```python
from build123d import *
from build123d.topology import SkipClean

# Parameters (mm, degrees)
SKETCH1_R            = 1.25
BRACKET_DEPTH        = 7.6
SKETCH2_R            = 1.5
ARM_DEPTH            = 1.6
SKETCH3_R            = 1.25
MOUNT_BLIND_DEPTH    = 1
EFFECTOR_START       = -5
SKETCH4_R            = 4
SKETCH4_R_2          = 1.5
EFFECTOR_MOUNT_DEPTH = 5
MOUNT_TRAP_DEPTH     = 2.4
SKETCH6_R            = 1.5
MOUNT_ADAPTOR_DEPTH  = 2.4
SKETCH7_W            = 12.99999996
SKETCH7_H            = 31.965
MIRROR_DELETE_DEPTH  = 37.150933583
ARM_SUPPORT_DEPTH    = 1.4
BODY_CHAMFER_SIZE    = 0.5
ARM_FILLET_R         = 0.5


with BuildPart() as part:
    # Sketch1 → Bracket (new body)
    with BuildSketch(Plane(origin=(0, 0, 0), x_dir=(1, 0, 0), z_dir=(0, 1, 0))):
        with BuildLine():
            Line((0, 7.765), (-9.4, 7.765))
            Line((-9.4, 7.765), (-12.531403257, 1.878614127))
            ThreePointArc((-12.531403257, 1.878614127), (-12.99999996, 0), (-12.531403257, -1.878614127))
            Line((-12.531403257, -1.878614127), (-9.4, -7.765))
            Line((-9.4, -7.765), (0, -7.765))
            Line((0, -7.765), (0, -5.765))
            ThreePointArc((0, -5.765), (-5.765, 0), (0, 5.765))
            Line((0, 5.765), (0, 7.765))
        make_face()
        with Locations(Location((-9, 0, 0), (0, 0, 90))):
            Circle(SKETCH1_R, mode=Mode.SUBTRACT)
    bracket = extrude(amount=BRACKET_DEPTH)

    # Sketch2 → Arm (add)
    with BuildSketch(Plane(origin=(-6.4, 0, 0), x_dir=(0, 0, -1), z_dir=(1, 0, 0))):
        with BuildLine():
            Line((-7.765, 0), (18.162978801, -15.342462002))
            ThreePointArc((18.162978801, -15.342462002), (24.160405232, -12.461418203), (19.2, -8.027016654))
            Line((19.2, -8.027016654), (7.765, 0))
            Line((7.765, 0), (-7.765, 0))
        make_face()
        with Locations((20.2, -11.9)):
            Circle(SKETCH2_R, mode=Mode.SUBTRACT)
    arm = extrude(amount=-ARM_DEPTH)

    # Sketch3 → Mount Blind (add)
    with BuildSketch(Plane.XZ):
        with Locations(Location((-9, 0, 0), (0, 0, 270))):
            Circle(SKETCH3_R)
    mount_blind = extrude(amount=-MOUNT_BLIND_DEPTH)

    # Sketch4 → Effector Mount (add)
    with SkipClean():  # the faces are left unmerged after this step: merging them gives an invalid solid
        with BuildSketch(Plane.ZY.offset(8).offset(EFFECTOR_START)):
            with Locations(Location((-20.2, -11.9, 0), (0, 0, 75.522487814))):
                Circle(SKETCH4_R)
            with Locations(Location((-20.2, -11.9, 0), (0, 0, 180))):
                Circle(SKETCH4_R_2, mode=Mode.SUBTRACT)
        effector_mount = extrude(amount=EFFECTOR_MOUNT_DEPTH)

    # Sketch5 → Mount Trap (cut)
    with SkipClean():  # the faces are left unmerged after this step: merging them gives an invalid solid
        with BuildSketch(Plane(origin=(-3, 0, 0), x_dir=(0, 0, -1), z_dir=(1, 0, 0))):
            Polygon((20.2, -8.724573519), (17.45, -10.31228676), (17.45, -13.48771324), (20.2, -15.075426481), (22.95, -13.48771324), (22.95, -10.31228676), align=None)
        mount_trap = extrude(amount=-MOUNT_TRAP_DEPTH, mode=Mode.SUBTRACT)

    # Sketch6 → Mount Adaptor (add)
    with SkipClean():  # the faces are left unmerged after this step: merging them gives an invalid solid
        with BuildSketch(Plane.ZY.offset(8)):
            Polygon((-17.45, -10.31228676), (-20.2, -8.724573519), (-22.95, -10.31228676), (-22.95, -13.48771324), (-20.2, -15.075426481), (-17.45, -13.48771324), align=None)
            with Locations(Location((-20.2, -11.9, 0), (0, 0, 180))):
                Circle(SKETCH6_R, mode=Mode.SUBTRACT)
        mount_adaptor = extrude(amount=MOUNT_ADAPTOR_DEPTH)

    # Mirror 2: Bracket, Arm, Mount Blind, Effector Mount, Mount Trap, Mount Adaptor across plane
    with SkipClean():  # the faces are left unmerged after this step: merging them gives an invalid solid
        add(bracket.mirror(Plane(origin=(0, 0, 0), x_dir=(0, 0, 1), z_dir=(1, 0, 0))))
        add(arm.mirror(Plane(origin=(0, 0, 0), x_dir=(0, 0, 1), z_dir=(1, 0, 0))))
        add(mount_blind.mirror(Plane(origin=(0, 0, 0), x_dir=(0, 0, 1), z_dir=(1, 0, 0))))
        add(effector_mount.mirror(Plane(origin=(0, 0, 0), x_dir=(0, 0, 1), z_dir=(1, 0, 0))))
        add(mount_trap.mirror(Plane(origin=(0, 0, 0), x_dir=(0, 0, 1), z_dir=(1, 0, 0))), mode=Mode.SUBTRACT)
        add(mount_adaptor.mirror(Plane(origin=(0, 0, 0), x_dir=(0, 0, 1), z_dir=(1, 0, 0))))

    # Sketch7 → Mirror Delete (cut, through all)
    with SkipClean():  # the faces are left unmerged after this step: merging them gives an invalid solid
        with BuildSketch(Plane(origin=(0, 7.6, 0), x_dir=(1, 0, 0), z_dir=(0, 1, 0))):
            with Locations((-6.49999998, 8.2175)):
                Rectangle(SKETCH7_W, SKETCH7_H)
        extrude(amount=-MIRROR_DELETE_DEPTH, mode=Mode.SUBTRACT)

    # Sketch8 → Arm Support (add)
    with SkipClean():  # the faces are left unmerged after this step: merging them gives an invalid solid
        with BuildSketch(Plane(origin=(8, 0, 0), x_dir=(0, 0, -1), z_dir=(1, 0, 0))):
            with BuildLine():
                Line((7.765, 0), (19.093373314, -7.952168015))
                ThreePointArc((19.093373314, -7.952168015), (16.218654953, -10.920769884), (17.388424851, -14.884132232))
                Line((17.388424851, -14.884132232), (-7.765, 0))
                Line((-7.765, 0), (7.765, 0))
            make_face()
        extrude(amount=ARM_SUPPORT_DEPTH)

    # Body Chamfer
    # the kernel refuses this chamfer: 0.5 mm, written as the material it takes off along each edge
    with BuildSketch(Plane(origin=(8.796100001, 0, -8.90020621), x_dir=(0.024274757051952575, 0.9996219169112968, -0.012913535559763734), z_dir=(0.4696535317878062, 0, 0.8828508141692119))) as body_chamfer_piece_1_section:
        Polygon((BODY_CHAMFER_SIZE * 0.999621916911, BODY_CHAMFER_SIZE * 0.0274958766106), (-BODY_CHAMFER_SIZE * 0.0274958766106, BODY_CHAMFER_SIZE * 0.999621916911), (0, 0), align=None)
    body_chamfer_piece_1 = extrude(amount=7.953316653, mode=Mode.PRIVATE)
    body_chamfer_piece_1 = split(body_chamfer_piece_1, bisect_by=Plane(origin=(9.4, 0.324892832, -7.480239841), z_dir=(1, 0, 0)), keep=Keep.TOP, mode=Mode.PRIVATE)
    add(body_chamfer_piece_1, mode=Mode.SUBTRACT)
    with BuildSketch(Plane(origin=(8.999999655, 0, 0), x_dir=(0.8828508331840651, 0, -0.4696534960438411), z_dir=(-0.4696534960438411, 0, -0.8828508331840651))) as body_chamfer_piece_2:
        Polygon((4.000000304, -BODY_CHAMFER_SIZE), (4.000000304 - BODY_CHAMFER_SIZE, 0), (4.000000304, 0), align=None)
    revolve(axis=Axis((8.999999655, 0, 0), (0, -1, 0)), revolution_arc=56.023613132, mode=Mode.SUBTRACT)
    with BuildSketch(Plane(origin=(12.531403257, 0, 1.878614127), x_dir=(0.02427475705195258, 0.9996219169112968, 0.012913535559763729), z_dir=(-0.46965353178780606, 0, 0.8828508141692119))) as body_chamfer_piece_3_section:
        Polygon((BODY_CHAMFER_SIZE * 0.999621916911, BODY_CHAMFER_SIZE * 0.0274958766106), (-BODY_CHAMFER_SIZE * 0.0274958766106, BODY_CHAMFER_SIZE * 0.999621916911), (0, 0), align=None)
    body_chamfer_piece_3 = extrude(amount=7.953316653, mode=Mode.PRIVATE)
    body_chamfer_piece_3 = split(body_chamfer_piece_3, bisect_by=Plane(origin=(9.4, 0.173767424, 5.065126353), z_dir=(1, 0, 0)), keep=Keep.TOP, mode=Mode.PRIVATE)
    add(body_chamfer_piece_3, mode=Mode.SUBTRACT)
    with BuildSketch(Plane(origin=(6.4, 0, 7.765), x_dir=(0, -0.02749587661058639, -0.9996219169112968), z_dir=(-1, 0, 0)), Plane(origin=(-1.285841494, 0, -7.765), x_dir=(0, -0.02749587661058639, 0.9996219169112968), z_dir=(1, 0, 0))) as body_chamfer_piece_4:
        Polygon((BODY_CHAMFER_SIZE * 0.999621916911, -BODY_CHAMFER_SIZE * 0.0274958766106), (-BODY_CHAMFER_SIZE * 0.0274958766106, -BODY_CHAMFER_SIZE * 0.999621916911), (0, 0), align=None)
    extrude(amount=7.685841494, mode=Mode.SUBTRACT)
    with BuildSketch(Plane(origin=(10.693671764, 0, 7.765), x_dir=(0, 0.9998167148671796, 0.019145147484436967), z_dir=(-1, 0, 0))) as body_chamfer_piece_5_section:
        Polygon((BODY_CHAMFER_SIZE * 0.999816714867, BODY_CHAMFER_SIZE * 0.0191451474844), (-BODY_CHAMFER_SIZE * 0.52563857146, BODY_CHAMFER_SIZE * 0.850707994669), (0, 0), align=None)
    body_chamfer_piece_5 = extrude(amount=2.693671764, mode=Mode.PRIVATE)
    body_chamfer_piece_5 = split(body_chamfer_piece_5, bisect_by=Plane(origin=(9.4, 0.125, 7.622443684), z_dir=(1, 0, 0)), keep=Keep.TOP, mode=Mode.PRIVATE)
    add(body_chamfer_piece_5, mode=Mode.SUBTRACT)

    # Arm Fillet
    arm_fillet_edges = [part.edges().sort_by_distance(p)[0] for p in [
        (7.2, 0, -7.765),
        (7.2, 0, 7.765),
    ]]
    fillet(arm_fillet_edges, radius=ARM_FILLET_R)


solid = part.part
```
Verification items for the finished model (mm, model axes). A direction names the side the tool comes from. Coordinates: 2 decimals unless noted, no trailing zeros. Write each loop counter-clockwise with the first axis right and the second up, starting at its lowest first coordinate (ties: lowest second). Pieces come first, ordered by that corner, then holes. Notation, with made-up numbers: M 17,64.25 L 71,64.25 A21 cw 71,84.25 Z; hole C -12.75,-6 d11. An arc over 180 degrees is marked long. Answer as a JSON object with one key per item and string values. Group by question number.
(1) Cross-section at B-B, the plane y = 3.25. Record the cut outline in (x, z) (3 decimals), and give its area (3 significant figures).
(2) Material ranges on line 1 (Y direction, x = 5.7, z = -20.2); line 2 (X direction, y = 5.75, z = 0) (3 decimals); line 3 (Z direction, x = 5.85, y = -11.9), recorded low to high.
(3) Cross-section at D-D, the plane y = -11.9. Record the cut outline in (x, z).
(4) Tool access check on faces 4 (the face through (5.4, -13.3, -18.9)), 5 (the face through (9.183, -14.27, -21.594)), 6 (the face through (6, 0, 0)), 7 (the face through (9, -12, -17.45)), 8 (the face through (9, 1, 0)). Record the directions out of +Z, -Z, +X, -X, +Y, -Y that give a thin tool (end or side, any length) a straight path to the whole face; none if there is none.
(5) Gauge pin test, flat ends, axial feed: pin 1 (3.5 mm diameter, centred on x = 3.5, y = 5.5, fed in from -Z) (3 decimals); pin 2 (1.9 mm diameter, centred on x = 9, y = -11, fed in from +Z); pin 3 (1.9 mm diameter, centred on x = 4.5, y = -12.5, fed in from +Z); pin 4 (1.9 mm diameter, centred on x = 4.5, z = -1, fed in from -Y). Record the tip position at first contact, or that the pin passes through.
(6) Cross-section at C-C, the plane x = 2.5. Record the cut outline in (y, z) (3 decimals), and give its area (3 significant figures).
(7) Release check for a two-part mould opening along Y. For faces 1 (the face through (13, 4, 0)), 2 (the face through (4, -12, -22.95)), 3 (the face through (10.726, 0.253, -4.747)) record: +Y half, -Y half, draft (parallel to the pull), parting line (faces both ways), or undercut.
(8) Cross-section at A-A, the plane x = 9. Record the cut outline in (y, z) (3 decimals), and give its area (3 significant figures).
Reply:
{
 "1": {"outline": "M 0,-7.765 L 9.4,-7.765 L 12.531,-1.879 A4 ccw 12.531,1.879 L 9.4,7.765 L 0,7.765 L 0,5.765 A5.765 cw 0,-5.765 Z; hole C 9,0 d2.5", "area": "120 mm²"},
 "2": {"line 1": "-15.9 to -13.4, -10.4 to -7.9", "line 2": "5.765 to 7.75, 10.25 to 13", "line 3": "-24.2 to -21.7, -18.7 to -16.2"},
 "3": {"outline": "M 3,-24.2 L 8,-24.2 L 8,-22.95 L 10.4,-22.95 L 10.4,-21.7 L 5.4,-21.7 L 5.4,-22.95 L 3,-22.95 Z; M 3,-17.45 L 5.4,-17.45 L 5.4,-18.7 L 10.4,-18.7 L 10.4,-17.45 L 8,-17.45 L 8,-16.1 L 9.4,-16.1 L 9.4,-12.35 L 6.4,-12.35 L 6.4,-16.2 L 3,-16.2 Z"},
 "4": {"face 4": "-X", "face 5": "-Z, +X, -Y", "face 6": "+Z, -Z, -X, -Y", "face 7": "+X, -Y", "face 8": "+Y"},
 "5": {"pin 1": "z = -7.765", "pin 2": "z = -9.22", "pin 3": "z = -16.2", "pin 4": "through"},
 "6": {"outline": "M 0,-7.265 L 0.5,-7.765 L 7.6,-7.765 L 7.6,-5.195 L 0,-5.195 Z; M 0,5.195 L 7.6,5.195 L 7.6,7.765 L 0.5,7.765 L 0,7.265 Z", "area": "38.8 mm²"},
 "7": {"face 1": "draft", "face 2": "undercut", "face 3": "-Y half"},
 "8": {"outline": "M -15.075,-20.2 L -13.488,-22.95 L -10.312,-22.95 L -8.725,-20.2 L -10.312,-17.45 L -13.488,-17.45 Z; M -14.884,-17.388 A4.1 cw -7.952,-19.093 L -0.149,-7.978 A0.5 cw 0.26,-7.765 L 7.6,-7.765 L 7.6,-1.25 L 1,-1.25 L 1,1.25 L 7.6,1.25 L 7.6,7.765 L 0.285,7.765 A0.5 ccw -0.145,7.52 Z; hole C -11.9,-20.2 d3", "area": "272 mm²"}
}
